Check sheet for the modelled part. Datum: model origin and axes. Units: mm. A direction names the side the tool comes from. Give positions to 0.01 mm unless a question says otherwise; leave off trailing zeros. Write each loop counter-clockwise with the first axis right and the second up, starting at its lowest first coordinate (ties: lowest second). Pieces come first, ordered by that corner, then holes. Notation, with made-up numbers: (-37, 42) -> (-33, 42) arc R17 ccw to (-33, 57) -> close; hole circle Ø8 at (83, 30). An arc over 180 degrees is marked (long way). Use a Markdown table: item, result. Add a question column.
1. Gauge pin test, flat end, axial feed: P1, Ø5, axis at y = -26.5, z = -5.5, coming from the +X side. Record the tip position at first contact, or that the pin passes through.
2. Scan lines: probe 1 along X at (y, z) = (4, -6.25); probe 2 along X at (y, z) = (-35.5, -2). Record each from-to range of solid material in increasing order. Write a range as [from, to].
3. Cross-section at B-B (y = 29.5). Enter the section's corners in (x, z), then the cut area to 3 significant figures.
4. Set-up check for faces 1 (the flat face through (31.75, 87, -8)), 2 (the flat face through (14.288, -49, -8)), 3 (the flat face through (15.875, -49, -8)): record each of +Z, -Z, +X, -X, +Y, -Y from which the full face is reachable in a straight line by a thin tool's end or side.
5. Cross-section at C-C (x = 20.75). Enter the section's corners in (y, z), then the cut area to 3 significant figures.
Autodesk Inventor part; units mm, degrees
ref_plane "YZ Plane" through (0, 0, 0) normal (1, 0, 0) x (0, 1, 0)
ref_plane "XZ Plane" through (0, 0, 0) normal (0, 1, 0) x (-1, 0, 0)
ref_plane "XY Plane" through (0, 0, 0) normal (0, 0, 1) x (1, 0, 0)
sketch "Sketch1" plane through (0, 0, 0) normal (0, 0, 1) x (1, 0, 0)
  line L0 (31.75, 85.8647) -> (31.75, 91.9353) construction
  line L1 (14.2875, -48.6156) -> (14.2875, -52.9844) construction
  line L2 (31.75, 94.2191) -> (31.75, 84.1662)
  line L3 (14.2875, -56.1455) -> (14.2875, -46.0925)
  line L4 (31.2464, 77.0306) -> (14.7911, -38.957)
  arc A0 (31.2464, 77.0306) -> (31.75, 84.1662) centre (-19.05, 84.1662) ccw
  arc A1 (14.7911, -38.957) -> (14.2875, -46.0925) centre (65.0875, -46.0925) ccw
  line L5 (33.3375, 94.2191) -> (33.3375, 84.1662)
  arc A2 (32.8181, 76.8076) -> (33.3375, 84.1662) centre (-19.05, 84.1662) ccw
  line L6 (32.8181, 76.8076) -> (16.3629, -39.1799)
  arc A3 (16.3629, -39.1799) -> (15.875, -46.0925) centre (65.0875, -46.0925) ccw
  line L7 (15.875, -46.0925) -> (15.875, -56.1455)
  line L8 (31.75, 94.2191) -> (33.3375, 94.2191)
  line L9 (14.2875, -56.1455) -> (15.875, -56.1455)
  line L10 (43.5527, 91.6185) -> (43.5527, 89.0199)
  point P0 (0, 0)
  dimension "d0" = 50.8
  dimension "d1" = 50.8
  dimension "d2" = 1.5875
  dimension "d26" = 2.5986
  dimension "d27" = 130.2587
  dimension "d28" = 10.053
extrude "Extrusion1" add sketch "Sketch1" against normal blind 12.7
fillet "Fillet1" radius 6.35 1 edges at (32.5437, 94.2191, 0)
fillet "Fillet2" radius 6.35 1 edges at (32.5437, 94.2191, -12.7)
fillet "Fillet3" radius 6.35 1 edges at (15.0812, -56.1455, 0)
fillet "Fillet4" radius 6.35 1 edges at (15.0812, -56.1455, -12.7)
sketch "Sketch2" plane through (33.3375, 84.1662, 0) normal (1, 0, 0) x (0, 0, -1)
  line L0 (12.7, 10.053) -> (12.7, 0) construction
  line L1 (0, 0) -> (0, 10.053) construction
  line L2 (0, 0) -> (12.7, 0) construction
  circle A0 centre (6.35, 4.7207) radius 6.35
  point P0 (0, -84.1662)
hole "Hole1" at (33.3375, 88.8868, -6.35) direction (-1, 0, 0) diameter 4.318 end through all
sketch "Sketch3" plane through (15.875, -56.1455, 0) normal (1, 0, 0) x (0, 0, -1)
  line L0 (12.7, 10.053) -> (12.7, 0) construction
  line L1 (0, 0) -> (0, 10.053) construction
  circle A0 centre (6.35, 5.3323) radius 6.35
  line L2 (0, 10.053) -> (12.7, 10.053) construction
  point P0 (0, 56.1455)
hole "Hole2" at (15.875, -50.8132, -6.35) direction (-1, 0, 0) diameter 4.318 end through all
properties part number "Endgame ramp polycarb"
Worked answers:
| question | item | result |
|---|---|---|
| 1 | P1 | stops at x = 18.52 |
| 2 | probe 1 | x = [20.89, 22.49] |
| 2 | probe 2 | x = [15.28, 16.88] |
| 3 | outline | (24.5, -12.7) -> (26.11, -12.7) -> (26.11, 0) -> (24.5, 0) -> close |
| 3 | area | 20.4 mm² |
| 4 | face 1 | +Z, -Z, -X, +Y |
| 4 | face 2 | +Z, -Z, -X, +Y, -Y |
| 4 | face 3 | +Z, -Z, +X, -Y |
| 5 | outline | (-8.26, -12.7) -> (3.05, -12.7) -> (3.05, 0) -> (-8.26, 0) -> close |
| 5 | area | 144 mm² |
